Can you work these out from the model? Positions are in its coordinate system, mm. Face numbers are marked on the shaded views. Round coordinates to 2 decimals unless told otherwise and drop trailing zeros. Write each loop counter-clockwise with the first axis right and the second up, starting at its lowest first coordinate (ties: lowest second). Pieces come first, ordered by that corner, then holes. Notation, with made-up numbers: (-19, 79) - (18, 79) arc R34 cw to (18, 109) - close; hole circle Ø2 at (59.25, 37). An arc over 180 degrees is marked (long way). One line per item, written item: value. Start each with the question number.
(1) If I drill on L1, parallel to Y at x = 12, z = 11.75; L2, parallel to X at y = -6.5, z = 9.5; L3, parallel to X at y = -4, z = 6.25, over which ranges is the centre line in solid material (lowest first)? Write a range as from..to.
(2) I want a section at C-C on x = 4. List the corners of the cut face in (y, z) for me, plus the area to 3 significant figures.
(3) I want a section at B-B on z = 4.75. List the corners of the cut face in (x, y) for me.
(4) Thinking about a two-plate mould opening in Y: for the marked faces 1, 2 and 3, which applies, +Y half, -Y half, draft (parallel to the pull), parting line (faces both ways), or undercut?
(5) I want a section at A-A on x = 0. List the corners of the cut face in (y, z) for me.
(6) I want a section at D-D on y = 6. List the corners of the cut face in (x, z) for me.
(7) I'm going to push flat-ended pins straight in: pin 1 Ø6.5 at (x, y) = (12, -5.593) entering from -Z; pin 2 Ø1.5 at (x, y) = (0, 6) entering from -Z. Where does each tip first touch, or does it pass through?
Autodesk Inventor part; units mm, degrees
ref_plane "YZ Plane" through (0, 0, 0) normal (1, 0, 0) x (0, 1, 0)
ref_plane "XZ Plane" through (0, 0, 0) normal (0, 1, 0) x (-1, 0, 0)
ref_plane "XY Plane" through (0, 0, 0) normal (0, 0, 1) x (1, 0, 0)
sketch "Sketch1" plane through (0, 0, 0) normal (0, 0, 1) x (1, 0, 0)
  line L0 (-20, 15) -> (20, 15)
  line L1 (20, 15) -> (20, -15)
  line L2 (20, -15) -> (-20, -15)
  line L3 (-20, -15) -> (-20, 15)
  point P0 (0, 0)
  point P1 (-20, 0)
  point P2 (0, 15)
  dimension "d0" = 30
  dimension "d1" = 40
extrude "Extrusion1" add sketch "Sketch1" along normal blind 15
sketch "Sketch2" plane through (-20, -15, 0) normal (-1, 0, 0) x (0, 0, 1)
  circle A0 centre (-3, 23) radius 5.15
  line L0 (0, 30) -> (0, 0)
  line L1 (0, 0) -> (15, 0)
  point P0 (0, 15)
  point P1 (0, 15)
  dimension "d5" = 10.3
  dimension "d17" = 23
  dimension "d18" = 3
extrude "Extrusion2" cut sketch "Sketch2" against normal through all
sketch "Sketch3" plane through (0, 0, 0) normal (0, 0, -1) x (-1, 0, 0)
  line L0 (-20, -15) -> (-20, 15)
  line L1 (-20, -15) -> (-20, 3.814)
  line L2 (20, -15) -> (-20, -15)
  line L3 (-20, 15) -> (20, 15)
  line L4 (20, 3.814) -> (20, -15)
  point P0 (0, 0)
  point P1 (-12, -5.593)
  point P2 (-20, 0)
  point P3 (-20, 12.186)
  point P4 (-20, -5.593)
  point P5 (0, 15)
  point P6 (0, -5.593)
  point P7 (12, -5.593)
  dimension "d19" = 8
  dimension "d20" = 8
hole "Hole1" at (12, -5.593, 0) at (0, -5.593, 0) at (-12, -5.593, 0) direction (0, 0, 1) diameter 5.5 end through all
properties part number "0008-10-011 Fixare AxaX Mijloc"
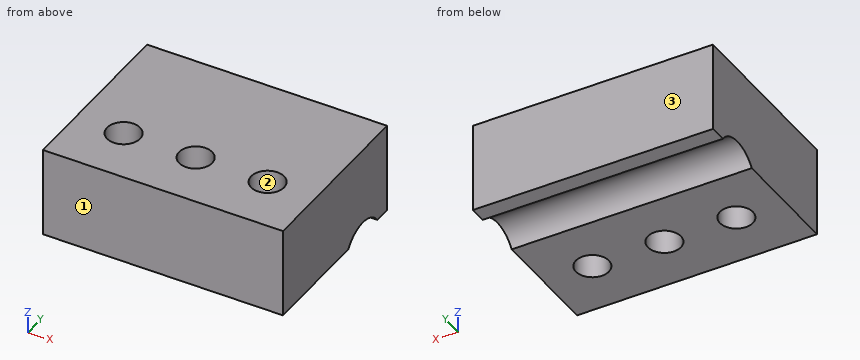
Established:
1. L1: -15..-8.34, -2.84..15
1. L2: -20..-14.6, -9.4..-2.6, 2.6..9.4, 14.6..20
1. L3: -20..-14.24, -9.76..-2.24, 2.24..9.76, 14.24..20
2. outline: (-15, 0) - (3.81, 0) arc R5.15 cw to (12.19, 0) - (15, 0) - (15, 15) - (-15, 15) - close
2. area: 437 mm2
3. outline: (-20, -15) - (20, -15) - (20, 15) - (-20, 15) - close; hole circle Ø5.5 at (-12, -5.59); hole circle Ø5.5 at (0, -5.59); hole circle Ø5.5 at (12, -5.59)
4. face 1: -Y half
4. face 2: undercut
4. face 3: +Y half
5. outline: (-15, 0) - (-8.34, 0) - (-8.34, 15) - (-15, 15) - close; (-2.84, 0) - (3.81, 0) arc R5.15 cw to (12.19, 0) - (15, 0) - (15, 15) - (-2.84, 15) - close
6. outline: (-20, 1.75) - (20, 1.75) - (20, 15) - (-20, 15) - close
7. pin 1: z = 0
7. pin 2: z = 1.35
